Check sheet for the modelled part. Datum: model origin and axes. Units: mm. A direction names the side the tool comes from. Round coordinates to 2 decimals unless told otherwise and drop trailing zeros. Write each loop counter-clockwise with the first axis right and the second up, starting at its lowest first coordinate (ties: lowest second). Pieces come first, ordered by that corner, then holes.
Item 1: Cross-section at B-B on z = 13.5. Enter the section's corners in (x, y), plus the area to 3 significant figures.
Item 2: Cross-section at D-D on z = -49.5. Enter the section's corners in (x, y), plus the area to 3 significant figures.
Item 3: Material ranges on line 1 (Y direction, x = 3, z = -50.5); line 2 (X direction, y = -0.25, z = -35); line 3 (X direction, y = -2.25, z = -15.5), recorded low to high.
Item 4: Go/stop test with flat-tipped pins: pin 1 Ø1.6 at (x, z) = (1, 54.5) entering from +Y; pin 2 Ø1.5 at (x, z) = (-2, 7.5) entering from -Y; pin 3 Ø2 at (x, z) = (-1.5, -2) entering from +Y. Record where each tip stops, or that it passes through.
Item 5: Cross-section at A-A on x = 0. Enter the section's corners in (y, z), plus the area to 3 significant figures.
Item 6: Tool access check on faces 1 (the flat face through (0, 3, -53)), 2 (the flat face through (0, 3, 53)), 3 (the cylindrical face through (-0.867, -3.905, 0.812)). Record the directions out of +Z, -Z, +X, -X, +Y, -Y that give a thin tool (end or side, any length) a straight path to the whole face; none if there is none.
Item 7: Cross-section at C-C on y = -1. Enter the section's corners in (x, z), plus the area to 3 significant figures.
from build123d import *

# Parameters (mm, degrees)
ESBO_O1_R                     = 4
RESSALTO_EXTRUS_O1_DEPTH      = 58
RESSALTO_EXTRUS_O1_DEPTH_BACK = 58
CORTE_EXTRUS_O1_DEPTH         = 10


with BuildPart() as part:
    # Esbo_o1 → Ressalto-extrus_o1 (new body, two sides)
    with BuildSketch(Plane.XY) as ressalto_extrus_o1_sk:
        Circle(ESBO_O1_R)
    extrude(amount=RESSALTO_EXTRUS_O1_DEPTH)
    extrude(ressalto_extrus_o1_sk.sketch, amount=-RESSALTO_EXTRUS_O1_DEPTH_BACK)

    # Esbo_o2 → Corte-extrus_o1 (cut)
    with BuildSketch(Plane.XY.offset(58)):
        with BuildLine():
            Line((2.645751311, 3), (-2.645751311, 3))
            ThreePointArc((-2.645751311, 3), (0, 4), (2.645751311, 3))
        make_face()
    corte_extrus_o1 = extrude(amount=-CORTE_EXTRUS_O1_DEPTH, mode=Mode.SUBTRACT)

    # Espelhar2: Corte-extrus_o1 across plane
    add(corte_extrus_o1.mirror(Plane.XY), mode=Mode.SUBTRACT)


solid = part.part
Response values:
1. outline: circle Ø8 at (0, 0)
1. area: 50.3 mm2
2. outline: (-2.65, 3) arc R4 ccw (long way) to (2.65, 3) - close
2. area: 46.6 mm2
3. line 1: y = -2.65 to 2.65
3. line 2: x = -3.99 to 3.99
3. line 3: x = -3.31 to 3.31
4. pin 1: stops at y = 3
4. pin 2: stops at y = -3.8
4. pin 3: stops at y = 3.97
5. outline: (-4, -58) - (3, -58) - (3, -48) - (4, -48) - (4, 48) - (3, 48) - (3, 58) - (-4, 58) - close
5. area: 908 mm2
6. face 1: -Z, +X, -X, +Y
6. face 2: +Z, +X, -X, +Y
6. face 3: +Z, -Z
7. outline: (-3.87, -58) - (3.87, -58) - (3.87, 58) - (-3.87, 58) - close
7. area: 899 mm2
